Geometry check sheet. Reference: the model listing, model coordinates, mm. Face numbers are marked on the shaded views. A direction names the side the tool comes from. Coordinates: 2 decimals unless noted, no trailing zeros. Loops run counter-clockwise (first coordinate to the right, second up) from the corner with the lowest first, then second, coordinate; pieces in that order, holes last. Notation, with made-up numbers: (-7, 61.25) -> (-3, 61.25) arc R18 ccw to (-3, 84.25) -> close; hole circle Ø4 at (37.25, 83). An arc over 180 degrees is marked (long way). Answer as a JSON object with one key per item and string values.
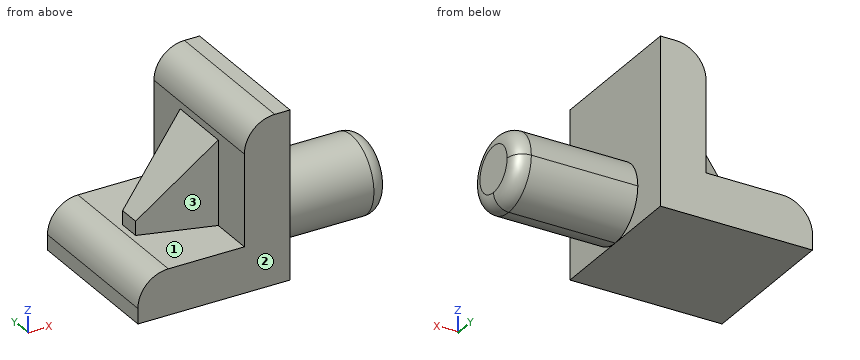
from build123d import *

# Parameters (mm, degrees)
F0_W        = 10
F0_H        = 10
F1_DEPTH    = 3
F3_DEPTH    = 8
F4_DEPTH    = 6
F5_T4_DEPTH = 27.5665061863
F6_R        = 2
F8_DEPTH    = 8
F9_R        = 1


# Not quite as in the source:
# - a fillet or chamfer that OpenCascade refuses, or shapes differently, is made with other operations: its cross-section is extruded or revolved along the edge and cut away or added


with BuildPart() as f1:
    # F0 (on Top) → F1 (new body)
    with BuildSketch(Plane.XY):
        with Locations((-5, -7.9495952278)):
            Rectangle(F0_W, F0_H)
    extrude(amount=F1_DEPTH)

    # F2 (on face) → F3 (join)
    with BuildSketch(Plane.XY.offset(3)):
        Polygon((0, -12.9495952278), (0, -2.9495952278), (-3, -2.9495952278), (-3, -5.8524622582), (-3, -7.9495952278), (-3, -10.0610805675), (-3, -12.9495952278), align=None)
    extrude(amount=F3_DEPTH)

    # F2 (on face) → F4 (join)
    with BuildSketch(Plane.XY.offset(3)):
        Polygon((-3, -7.9495952278), (-3, -5.8524622582), (-7.6078968298, -7.2329440242), (-7.6078968298, -8.6711510528), (-3, -10.0610805675), align=None)
    extrude(amount=F4_DEPTH)

    # F5: chamfer of 5.08 on 1 edges, made by hand


with BuildPart() as f5_tool2:
    # F5_s3 → F5_t4 (new body)
    with BuildSketch(Plane.XZ.offset(-5.8312055546)):
        Polygon((-7.6078968298, 3.92), (-2.5278968298, 9), (-7.6078968298, 9), align=None)
    extrude(amount=F5_T4_DEPTH)

    split(bisect_by=Plane.YZ.offset(-3), keep=Keep.BOTTOM)


with BuildPart() as f1_1:
    add(f1.part)

    # F5_t1: cut F5_tool2
    add(f5_tool2.part, mode=Mode.SUBTRACT)

    # F6
    f6_edges = [f1_1.edges().sort_by_distance(p)[0] for p in [
        (-10, -7.949595, 3),
        (-3, -7.949595, 11),
    ]]
    fillet(f6_edges, radius=F6_R)

    # F7 (on face) → F8 (join)
    with BuildSketch(Plane.YZ):
        with BuildLine():
            ThreePointArc((-7.9495952278, 0), (-6.1818282749, 0.732233047), (-5.4495952278, 2.5))
            ThreePointArc((-5.4495952278, 2.5), (-9.7173621808, 4.267766953), (-7.9495952278, 0))
        make_face()
    extrude(amount=F8_DEPTH)

    # F9
    f9_edges = [f1_1.edges().sort_by_distance(p)[0] for p in [
        (8, -7.949595, 5),
    ]]
    fillet(f9_edges, radius=F9_R)


solid = f1_1.part
1. Depth check by flat-ended pin: P1, Ø4, axis at x = -6, z = 5.5, coming from the -Y side; P2, Ø6, axis at x = -6.5, y = -6, coming from the +Z side; P3, Ø3, axis at y = -9, z = 6, coming from the -X side. Enter the tip coordinate at first touch or a pass-through.
Evaluation:
{"P1": "stops at y = -9.76", "P2": "stops at z = 8.03", "P3": "stops at x = -7.02"}
2. Thickness scan on probe 1 along X at (y, z) = (-8.25, 9); probe 2 along Y at (x, z) = (6.5, 4.5); probe 3 along Z at (x, y) = (-7.75, -4.5). Record the ranges inside material, lowest first. Write a range as from..to.
Evaluation:
{"probe 1": "x = -3..0", "probe 2": "y = -9.45..-6.45", "probe 3": "z = 0..3"}
3. Tool access check on the marked faces 1, 2 and 3. Record the directions out of +Z, -Z, +X, -X, +Y, -Y that give a thin tool (end or side, any length) a straight path to the whole face; none if there is none.
Evaluation:
{"face 1": "+Z, -X", "face 2": "+Z, -Z, +X, -X, -Y", "face 3": "+Z, -X, -Y"}
4. Section check C-C, the plane x = 2.75. Record the boundary of the cut face in (y, z), then the cut area to 3 significant figures.
Evaluation:
{"outline": "circle Ø5 at (-7.95, 2.5)", "area": "19.6 mm^2"}
5. Section check A-A, the plane y = -3.75. Record the boundary of the cut face in (x, z), then the cut area to 3 significant figures.
Evaluation:
{"outline": "(-10, 0) -> (0, 0) -> (0, 11) -> (-1, 11) arc R2 ccw to (-3, 9) -> (-3, 3) -> (-8, 3) arc R2 ccw to (-10, 1) -> close", "area": "52.3 mm^2"}
6. Section check B-B, the plane z = 5.5. Record the boundary of the cut face in (x, y), then the cut area to 3 significant figures.
Evaluation:
{"outline": "(-6.03, -9.15) -> (-3, -10.06) -> (-3, -12.95) -> (0, -12.95) -> (0, -2.95) -> (-3, -2.95) -> (-3, -5.85) -> (-6.03, -6.76) -> close", "area": "40.0 mm^2"}
7. Section check D-D, the plane z = 10. Record the boundary of the cut face in (x, y), then the cut area to 3 significant figures.
Evaluation:
{"outline": "(-2.73, -12.95) -> (0, -12.95) -> (0, -2.95) -> (-2.73, -2.95) -> close", "area": "27.3 mm^2"}
